Input: part model. Units: mm. Frame: model coordinates. Face numbers are marked on the shaded views. A direction names the side the tool comes from. Round coordinates to 2 decimals unless told otherwise and drop trailing zeros. Loops run counter-clockwise (first coordinate to the right, second up) from the corner with the lowest first, then second, coordinate; pieces in that order, holes last. Notation, with made-up numbers: M -30.5,-35.5 L -0.5,-35.5 A25 ccw -0.5,-12.5 Z; hole C 57.25,39.5 d10. An arc over 180 degrees is marked long. Put each result on its own line as item: value. Start each with the question number.
1) Section A-A on x = 25. Output: boundary loops of the cut face in (y, z).
2) Line query: probe 1 along X at (y, z) = (-5.75, 1); probe 2 along Z at (x, y) = (17.5, 0.25); probe 3 along X at (y, z) = (8, -2.5). Output: solid intervals per line, ascending.
3) Draft query along X for the marked faces 1, 2 and 3. Return one class per face: +X half, -X half, draft (parallel to the pull), parting line (faces both ways), or undercut.
4) Reachability of the marked faces 4, 5 and 6 from +Z, -Z, +X, -X, +Y, -Y: full face, straight path, thin tool, end or side. Return the list, or none.
5) Pin query (flat end, axial travel): pin 1 (1.7 mm diameter, centred on y = -1, z = 2, fed in from -X); pin 2 (2 mm diameter, centred on x = 25, y = 3, fed in from -Z); pin 3 (6 mm diameter, centred on x = 24, y = 7, fed in from +Z). Return the tip coordinate at first contact, or that it passes through.
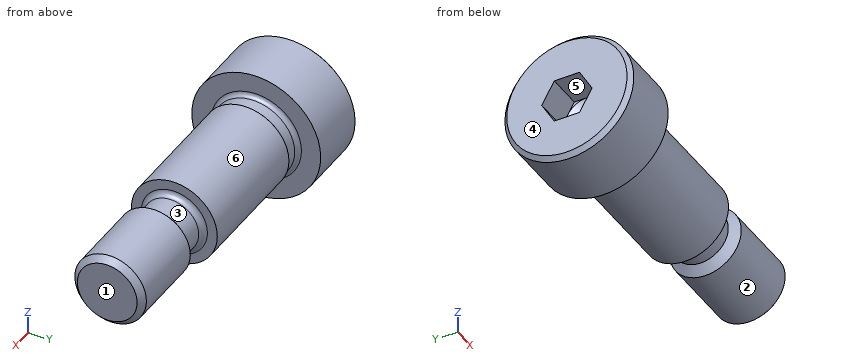
from build123d import *

# Parameters (mm, degrees)
CHAMFER1_SIZE = 0.6
HEX_2_DEPTH   = 4.9


with BuildPart() as part:
    # BodySke → BaseBody (revolve)
    with BuildSketch(Plane.XY):
        with BuildLine():
            Line((0, 0), (0, 9))
            Line((0, 9), (9, 9))
            Line((9, 9), (9, 6.31))
            ThreePointArc((9, 6.31), (9.175735931, 5.885735931), (9.6, 5.71))
            Line((9.6, 5.71), (11.218, 5.71))
            Line((11.218, 5.71), (11.5, 5.992))
            Line((11.5, 5.992), (29, 5.992))
            Line((29, 5.992), (29, 4.615))
            ThreePointArc((29, 4.615), (29.225527778, 4.070527778), (29.77, 3.845))
            Line((29.77, 3.845), (32.7, 3.845))
            Line((32.7, 3.845), (33.855, 5))
            Line((33.855, 5), (44.572, 5))
            Line((44.572, 5), (45.4, 4.172))
            Line((45.4, 4.172), (45.4, 0))
            Line((45.4, 0), (0, 0))
        make_face()
    revolve(axis=Axis((-6.35, 0, 0), (1, 0, 0)))

    # Chamfer1
    chamfer1_edges = [part.edges().sort_by_distance(p)[0] for p in [
        (0, -9, 0),
    ]]
    chamfer(chamfer1_edges, length=CHAMFER1_SIZE)

    # Sketch2 → PreBroach (revolve, cut)
    with BuildSketch(Plane.XY):
        Polygon((0, 3.0475), (4.9, 3.0475), (6.659474945, 0), (0, 0), align=None)
    revolve(axis=Axis((0, 0, 0), (1, 0, 0)), mode=Mode.SUBTRACT)

    # Sketch3 → Hex 2 (cut)
    with BuildSketch(Plane.ZY):
        Polygon((-3.0475, -1.759474945), (-3.0475, 1.759474945), (0, 3.518949891), (3.0475, 1.759474945), (3.0475, -1.759474945), (0, -3.518949891), align=None)
    extrude(amount=-HEX_2_DEPTH, mode=Mode.SUBTRACT)


solid = part.part
Geometry results:
1. outline: C 0,0 d11.98
2. probe 1: x = 0 to 9.23, 11.34 to 29
2. probe 2: z = -5.99 to 5.99
2. probe 3: x = 0 to 9
3. face 1: +X half
3. face 2: draft
3. face 3: undercut
4. face 4: +Z, -Z, -X, +Y, -Y
4. face 5: -X
4. face 6: +X
5. pin 1: stops at x = 4.9
5. pin 2: stops at z = -5.65
5. pin 3: stops at z = 4.46
